Check sheet for the modelled part. Datum: model origin and axes. Units: mm. A direction names the side the tool comes from. Round coordinates to 2 decimals unless told otherwise and drop trailing zeros. Loops run counter-clockwise (first coordinate to the right, second up) from the corner with the lowest first, then second, coordinate; pieces in that order, holes last. Notation, with made-up numbers: (22.25, 50.25) - (62.25, 50.25) arc R27 ccw to (62.25, 74.25) - close; hole circle Ø3 at (-40, -20). An arc over 180 degrees is marked (long way). Answer in a Markdown table with one row per item. Add a question column.
(1) Access from +Z, -Z, +X, -X, +Y, -Y to the whole of each face (thin tool, end or side, straight path). Record for faces 1 (the cylindrical face through (-13.77, -125.22, 61.99)), 2 (the flat face through (-1, -254, -1)).
(2) Cross-section at A-A on x = 0. Enter the section's corners in (y, z).
(3) Cross-section at C-C on y = -18. Enter the section's corners in (x, z).
(4) Gauge pin test, flat ends, axial feed: pin 1 (2 mm diameter, centred on y = -204, z = -18, fed in from +X); pin 2 (6 mm diameter, centred on x = 36, y = -167.5, fed in from -Z); pin 3 (1.5 mm diameter, centred on x = -27.5, y = -198.5, fed in from -Z). Record the tip position at first contact, or that the pin passes through.
(5) Thickness scan on line 1 along Y through (x, z) = (-30.5, 78); line 2 along X through (y, z) = (-35, 0); line 3 along X through (y, z) = (-145.5, 37). Record the ranges inside material, lowest first.
(6) Cross-section at B-B on z = -53.5. Enter the section's corners in (x, y).
(7) Cross-section at D-D on y = 78.5. Enter the section's corners in (x, z), then the cut area to 3 significant figures.
from build123d import *

# Parameters (mm, degrees)
SKETCH1_R           = 63.5
BOSS_EXTRUDE1_DEPTH = 254
BOSS_EXTRUDE2_DEPTH = 101.6


with BuildPart() as part:
    # Sketch1 → Boss-Extrude1 (new body)
    with BuildSketch(Plane(origin=(0, 0, 0), x_dir=(1, 0, 0), z_dir=(0, 1, 0))):
        Circle(SKETCH1_R)
    extrude(amount=-BOSS_EXTRUDE1_DEPTH)

    # Sketch2 → Boss-Extrude2 (add)
    with BuildSketch(Plane(origin=(0, 0, 0), x_dir=(1, 0, 0), z_dir=(0, 1, 0))):
        Polygon((-50.613670356, 87.665448614), (50.613670356, 87.665448614), (101.227340712, 0), (50.613670356, -87.665448614), (-50.613670356, -87.665448614), (-101.227340712, 0), align=None)
    extrude(amount=BOSS_EXTRUDE2_DEPTH)


solid = part.part
Answers:
| question | item | result |
|---|---|---|
| 1 | face 1 | -Y |
| 1 | face 2 | +Z, -Z, +X, -X, -Y |
| 2 | outline | (-254, -63.5) - (0, -63.5) - (0, -87.67) - (101.6, -87.67) - (101.6, 87.67) - (0, 87.67) - (0, 63.5) - (-254, 63.5) - close |
| 3 | outline | circle Ø127 at (0, 0) |
| 4 | pin 1 | stops at x = 61.18 |
| 4 | pin 2 | stops at z = -54.25 |
| 4 | pin 3 | stops at z = -57.59 |
| 5 | line 1 | y = 0 to 101.6 |
| 5 | line 2 | x = -63.5 to 63.5 |
| 5 | line 3 | x = -51.61 to 51.61 |
| 6 | outline | (-70.34, 0) - (-34.21, 0) - (-34.21, -254) - (34.21, -254) - (34.21, 0) - (70.34, 0) - (70.34, 101.6) - (-70.34, 101.6) - close |
| 7 | outline | (-101.23, 0) - (-50.61, -87.67) - (50.61, -87.67) - (101.23, 0) - (50.61, 87.67) - (-50.61, 87.67) - close |
| 7 | area | 26,600 mm^2 |
